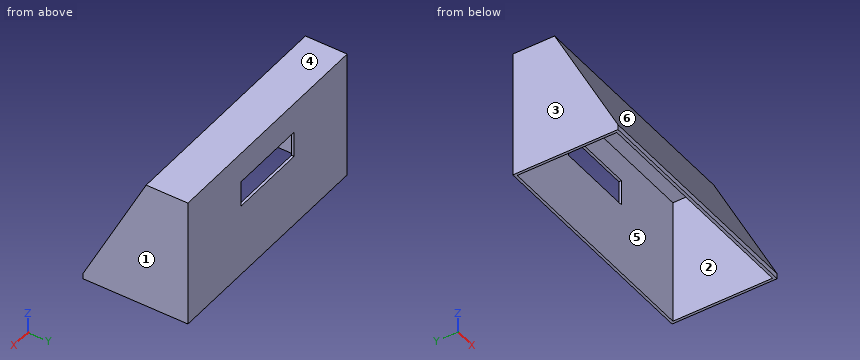
Autodesk Fusion 360 part; units mm, degrees
sketch "Unsorted Smarties Holder" plane through (0, 0, 0) normal (1, 0, 0) x (0, 1, 0)
  line L0 (0, 0) -> (93.3717, 0)
  line L1 (93.3717, 0) -> (93.3717, 143.115)
  line L2 (93.3717, 143.115) -> (45.2924, 143.115)
  line L3 (45.2924, 143.115) -> (-27.6283, 0)
  line L4 (-27.6283, 0) -> (0, 0)
  line L5 (-27.6283, 0) -> (93.3717, 0)
  line L6 (93.3717, 0) -> (93.3717, -6)
  line L7 (93.3717, -6) -> (-27.6283, -6)
  line L8 (-27.6283, -6) -> (-27.6283, 0)
  dimension "d5" = 143.115
  dimension "d14" = 63
  dimension "d23" = 121
  dimension "d31" = 6
extrude "Extrude1" add sketch "Unsorted Smarties Holder" along normal blind 270
sketch "Sketch3" plane through (270, 0, 0) normal (1, 0, 0) x (0, 1, 0)
  line L0 (93.3717, -6) -> (93.3717, 143.115)
  line L1 (93.3717, 143.115) -> (45.2924, 143.115)
  line L2 (45.2924, 143.115) -> (-27.6283, 0)
  line L3 (90.3717, 140.115) -> (90.3717, 0)
  line L4 (90.3717, 0) -> (-24.2614, 0)
  line L5 (-24.2614, 0) -> (47.1308, 140.115)
  line L6 (47.1308, 140.115) -> (90.3717, 140.115)
  line L7 (-27.6283, 0) -> (-27.6283, -6)
  line L8 (-27.6283, -6) -> (93.3717, -6)
  line L9 (-24.2614, 0) -> (90.3717, 0)
  line L10 (90.3717, 0) -> (90.3717, -6)
  line L11 (90.3717, -6) -> (-24.2614, -6)
  line L12 (-24.2614, -6) -> (-24.2614, 0)
  dimension "d15" = 3
  dimension "d16" = 3
  dimension "d17" = 3
  dimension "d18" = 3
  dimension "d32" = 6
  dimension "d33" = 6
extrude "Extrude3" cut sketch "Sketch3" against normal blind 264 from surface at -3 contours L4 L8 L9 L10 L11 L12 | L3 L4 L5 L6 L9
sketch "Smarties Feed" plane through (0, 93.3717, 0) normal (0, 1, 0) x (-1, 0, 0)
  line L0 (0, -6) -> (0, 143.115)
  line L1 (0, 143.115) -> (-270, 143.115)
  line L2 (-270, 143.115) -> (-270, -6)
  line L3 (-180, 108.115) -> (-90, 108.115)
  line L4 (-90, 108.115) -> (-90, 78.115)
  line L5 (-90, 78.115) -> (-180, 78.115)
  line L6 (-180, 78.115) -> (-180, 108.115)
  line L7 (-270, -6) -> (0, -6)
  dimension "d24" = 30
  dimension "d25" = 90
  dimension "d26" = 90
  dimension "d27" = 90
  dimension "d28" = 35
extrude "Extrude4" cut sketch "Smarties Feed" against normal blind 3 contours L3 L4 L5 L6
equation "polycarbonateThickness = 3 mm"
equation "d14 = 180 deg - 117 deg"
equation "d15 = polycarbonateThickness"
equation "d16 = polycarbonateThickness"
equation "d17 = polycarbonateThickness"
equation "d18 = polycarbonateThickness"
equation "d21 = -( 270 mm - 2 * polycarbonateThickness )"
equation "d28 = 41 mm - 6 mm"
Geometry: final body of the model. Coordinates: model frame, mm. Face numbers are marked on the shaded views. A direction names the side the tool comes from. Coordinates: 2 decimals unless noted, no trailing zeros. Order: outer loops, then holes, each group sorted by start corner. A loop starts at its lowest first (then second) coordinate and runs counter-clockwise, first axis right, second up.
(1) Draft query along X for the marked faces 1, 2, 3 and 4. Return one class per face: pulls with the +X half, pulls with the -X half, needs draft (parallel to the pull), parting line crosses it, or undercut.
(2) First-contact query: pin 1 (10 mm diameter, centred on x = 118, z = 58.5, fed in from -Y); pin 2 (10 mm diameter, centred on x = 75, y = 42.5, fed in from -Z); pin 3 (10 mm diameter, centred on x = 231.5, y = 3, fed in from -Z). Flat tips, straight axial feed; report the tip coordinate or a pass-through.
(3) Access query for the marked faces 5 and 6. Directions: +Z, -Z, +X, -X, +Y, -Y. A direction counts if a zero-diameter tool reaches every point of the face in a straight line with its end or side. Return the directions, or none.
(4) Section query C-C (z = 115.5). Return the cut outline in (x, y), plus the area to 3 significant figures.
(5) Material intervals for probe 1 along X at (y, z) = (81, 117.5); probe 2 along Z at (x, y) = (23, 75) (3 decimals); probe 3 along Y at (x, z) = (240, 76), sorted ascending.
(6) Section query D-D (x = 76). Return the cut outline in (y, z) (3 decimals), plus the area to 3 significant figures.
(7) Section query B-B (x = 103.5). Return the cut outline in (y, z) (3 decimals).
(8) Section query A-A (y = 58.5). Return the cut outline in (x, z) (3 decimals).
Solution:
1. face 1: pulls with the +X half
1. face 2: undercut
1. face 3: pulls with the -X half
1. face 4: needs draft
2. pin 1: stops at y = -0.37
2. pin 2: stops at z = 121.21
2. pin 3: stops at z = 43.69
3. face 5: -Z
3. face 6: +Z, +X, -X, -Y
4. outline: (0, 31.22) - (270, 31.22) - (270, 93.37) - (0, 93.37) - close; hole (3, 34.59) - (267, 34.59) - (267, 90.37) - (3, 90.37) - close
4. area: 2,050 mm2
5. probe 1: x = 0 to 3, 267 to 270
5. probe 2: z = 140.115 to 143.115
5. probe 3: y = 11.1 to 14.46, 90.37 to 93.37
6. outline: (-27.628, -6) - (-24.261, -6) - (-24.261, 0) - (47.131, 140.115) - (90.372, 140.115) - (90.372, -6) - (93.372, -6) - (93.372, 143.115) - (45.292, 143.115) - (-27.628, 0) - close
6. area: 1,080 mm2
7. outline: (-27.628, -6) - (-24.261, -6) - (-24.261, 0) - (47.131, 140.115) - (90.372, 140.115) - (90.372, 108.115) - (93.372, 108.115) - (93.372, 143.115) - (45.292, 143.115) - (-27.628, 0) - close; (90.372, -6) - (93.372, -6) - (93.372, 78.115) - (90.372, 78.115) - close
8. outline: (0, -6) - (3, -6) - (3, 140.115) - (267, 140.115) - (267, -6) - (270, -6) - (270, 143.115) - (0, 143.115) - close
